Input: dimensioned drawing with shaded views. Units: mm. Origin: part minimum x, y, z. A direction names the side the tool comes from. Coordinates: 2 decimals unless noted, no trailing zeros. Order: outer loops, then holes, each group sorted by start corner. A loop starts at its lowest first (then second) coordinate and runs counter-clockwise, first axis right, second up.
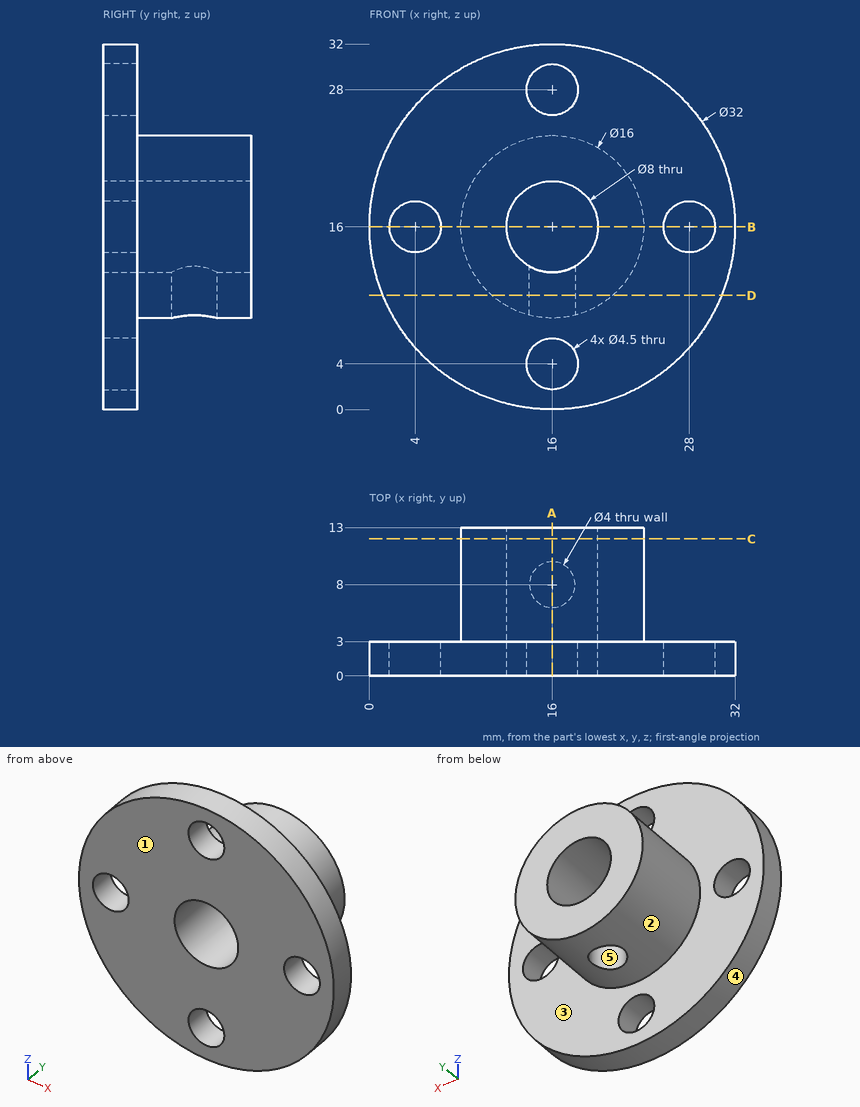
1. Draft query along Y for the marked faces 3, 4 and 5. Return one class per face: released by +Y, released by -Y, zero draft, split by the parting line, or undercut.
Findings:
face 3: released by +Y
face 4: zero draft
face 5: undercut
2. Access query for the marked faces 1 and 2. Directions: +Z, -Z, +X, -X, +Y, -Y. A direction counts if a zero-diameter tool reaches every point of the face in a straight line with its end or side. Return the directions, or none.
Findings:
face 1: +Z, -Z, +X, -X, -Y
face 2: +Y
3. Section query C-C on y = 12. Return loops of the section in (x, z), plus the area to 3 significant figures.
Findings:
outline: circle Ø16 at (16, 16); hole circle Ø8 at (16, 16)
area: 151 mm2
4. Section query B-B on z = 16. Return loops of the section in (x, y), plus the area to 3 significant figures.
Findings:
outline: (0, 0) - (1.75, 0) - (1.75, 3) - (0, 3) - close; (6.25, 0) - (12, 0) - (12, 13) - (8, 13) - (8, 3) - (6.25, 3) - close; (20, 0) - (25.75, 0) - (25.75, 3) - (24, 3) - (24, 13) - (20, 13) - close; (30.25, 0) - (32, 0) - (32, 3) - (30.25, 3) - close
area: 125 mm2
5. Pin query (flat end, axial travel): P1, Ø2.5, axis at x = 16, y = 8, coming from the -Z side; P2, Ø1, axis at x = 13, y = 5.5, coming from the +Z side; P3, Ø7, axis at x = 4, z = 16, coming from the +Y side. Return the tip coordinate at first contact, or that it passes through.
Findings:
P1: stops at z = 19.8
P2: stops at z = 23.6
P3: stops at y = 3
6. Section query D-D on z = 10. Return loops of the section in (x, y), plus the area to 3 significant figures.
Findings:
outline: (1.17, 0) - (30.83, 0) - (30.83, 3) - (21.29, 3) - (21.29, 13) - (10.71, 13) - (10.71, 3) - (1.17, 3) - close; hole circle Ø4 at (16, 8)
area: 182 mm2
7. Ray query, line 1 (X direction, y = 1.65, z = 16); line 2 (Y direction, x = 12, z = 6); line 3 (Z direction, x = 16.5, y = 10.5). Return the intervals inside material, ascending.
Findings:
line 1: x = 0 to 1.75, 6.25 to 12, 20 to 25.75, 30.25 to 32
line 2: y = 0 to 3
line 3: z = 8.02 to 12.03, 19.97 to 23.98
8. Section query A-A on x = 16. Return loops of the section in (y, z), plus the area to 3 significant figures.
Findings:
outline: (0, 0) - (3, 0) - (3, 1.75) - (0, 1.75) - close; (0, 6.25) - (3, 6.25) - (3, 8) - (6, 8) - (6, 12) - (0, 12) - close; (0, 20) - (13, 20) - (13, 24) - (3, 24) - (3, 25.75) - (0, 25.75) - close; (0, 30.25) - (3, 30.25) - (3, 32) - (0, 32) - close; (10, 8) - (13, 8) - (13, 12) - (10, 12) - close
area: 109 mm2
